Build history of the part. All positions in model axes, mm. A direction names the side the tool comes from. Coordinates: 2 decimals unless noted, no trailing zeros. Write each loop counter-clockwise with the first axis right and the second up, starting at its lowest first coordinate (ties: lowest second). Pieces come first, ordered by that corner, then holes.
from build123d import *

# Parameters (mm, degrees)
BASESKETCH_R              = 137.5
BASE_DEPTH                = 15
MOUNTINGHOLES_R           = 3.25
CUT_EXTRUDE1_DEPTH        = 15
BEARINGJ1_R               = 25
CUT_EXTRUDE3_DEPTH        = 15
CUT_EXTRUDE4_START        = 15
BEARINGRADIALCONSTRAINT_R = 30
CUT_EXTRUDE4_DEPTH        = 5


with BuildPart() as part:
    # BaseSketch → Base (new body)
    with BuildSketch(Plane(origin=(0, 0, 0), x_dir=(1, 0, 0), z_dir=(0, 1, 0))):
        Circle(BASESKETCH_R)
    extrude(amount=BASE_DEPTH)

    # MountingHoles → Cut-Extrude1 (cut)
    with BuildSketch(Plane(origin=(0, 0, 0), x_dir=(1, 0, 0), z_dir=(0, 1, 0))):
        with Locations((-80, 95)):
            Circle(MOUNTINGHOLES_R)
        with Locations((-80, -95)):
            Circle(MOUNTINGHOLES_R)
        with Locations((80, -95)):
            Circle(MOUNTINGHOLES_R)
        with Locations((80, 95)):
            Circle(MOUNTINGHOLES_R)
    extrude(amount=CUT_EXTRUDE1_DEPTH, mode=Mode.SUBTRACT)

    # BearingJ1 → Cut-Extrude3 (cut)
    with BuildSketch(Plane(origin=(0, 0, 0), x_dir=(1, 0, 0), z_dir=(0, 1, 0))):
        Circle(BEARINGJ1_R)
    extrude(amount=CUT_EXTRUDE3_DEPTH, mode=Mode.SUBTRACT)

    # BearingRadialConstraint → Cut-Extrude4 (cut)
    with BuildSketch(Plane(origin=(0, 0, 0), x_dir=(1, 0, 0), z_dir=(0, 1, 0)).offset(CUT_EXTRUDE4_START)):
        Circle(BEARINGRADIALCONSTRAINT_R)
    extrude(amount=-CUT_EXTRUDE4_DEPTH, mode=Mode.SUBTRACT)


solid = part.part
(1) Flat gauge pins, fed straight in: P1, Ø6, axis at y = 10, z = -94, coming from the +X side; P2, Ø2, axis at y = 10, z = 23.5, coming from the -X side; P3, Ø8, axis at y = 9, z = -41, coming from the +X side. Where does each tip first touch, or does it go through?
(2) Slice it at D-D, the plane x = 80. List the corners of the cut face in (y, z).
(3) Slice it at C-C, the plane y = 5.5. List the corners of the cut face in (x, z).
(4) Slice it at A-A, the plane z = 0. List the corners of the cut face in (x, y).
(5) Probe L1, parallel to X at y = 5.5, z = -95; L2, parallel to Z at x = -80, y = 3.5; L3, parallel to Z at x = 0, y = 11.55. List the from-to ranges inside material, lowest first.
(6) Two-plate mould, pull along X, no slides. Class faces 1 (the cylindrical face through (79.295, 7.395, 98.173)), 2 (the cylindrical face through (131.15, 7.4, -41.3)), 3 (the flat face through (-2, 0, 29)): pulls with the +X half, pulls with the -X half, needs draft (parallel to the pull), parting line crosses it, or undercut.
(7) 3-axis set-ups, long thin cutter, end or side, ignore diameter. For faces 4 (the flat face through (-2, 15, -32)), 5 (the cylindrical face through (-29.97, 12.54, -1.32)): which of +Z, -Z, +X, -X, +Y, -Y reach the whole face in a straight line?
(8) Slice it at B-B, the plane x = 0. List the corners of the cut face in (y, z).
Results:
1. P1: stops at x = 103.08
1. P2: stops at x = -135.65
1. P3: stops at x = 132.43
2. outline: (0, -111.83) - (15, -111.83) - (15, -98.25) - (0, -98.25) - close; (0, -91.75) - (15, -91.75) - (15, 91.75) - (0, 91.75) - close; (0, 98.25) - (15, 98.25) - (15, 111.83) - (0, 111.83) - close
3. outline: circle Ø275 at (0, 0); hole circle Ø6.5 at (-80, -95); hole circle Ø6.5 at (-80, 95); hole circle Ø50 at (0, 0); hole circle Ø6.5 at (80, -95); hole circle Ø6.5 at (80, 95)
4. outline: (-137.5, 0) - (-25, 0) - (-25, 10) - (-30, 10) - (-30, 15) - (-137.5, 15) - close; (25, 0) - (137.5, 0) - (137.5, 15) - (30, 15) - (30, 10) - (25, 10) - close
5. L1: x = -99.4 to -83.25, -76.75 to 76.75, 83.25 to 99.4
5. L2: z = -111.83 to -98.25, -91.75 to 91.75, 98.25 to 111.83
5. L3: z = -137.5 to -30, 30 to 137.5
6. face 1: undercut
6. face 2: parting line crosses it
6. face 3: needs draft
7. face 4: +Z, -Z, +X, -X, +Y
7. face 5: +Y
8. outline: (0, -137.5) - (15, -137.5) - (15, -30) - (10, -30) - (10, -25) - (0, -25) - close; (0, 25) - (10, 25) - (10, 30) - (15, 30) - (15, 137.5) - (0, 137.5) - close
